```python
from build123d import *

# Parameters (mm, degrees)
SKETCH_1_R           = 1.7
EXTRUDE_1_DEPTH      = 4
EXTRUDE_2_DEPTH      = 4
EXTRUDE_2_DEPTH_BACK = 4


with BuildPart() as part:
    # Sketch 1 → Extrude 1 (new body)
    with BuildSketch(Plane(origin=(0, 0, 0), x_dir=(1, 0, 0), z_dir=(0, 1, 0))):
        with BuildLine():
            Line((0, -50), (0, -43))
            add(Edge.make_bspline(
                [(-10.000145873, 27.475174978), (-27.697978685, -43), (0, -43)],
                knots=[4.019246634, 4.019246634, 4.019246634, 6.283185307, 6.283185307, 6.283185307], degree=2, weights=[1, 0.42487789, 1]))
            ThreePointArc((-10.000145873, 27.475174978), (-18.360814479, 27.113576543), (-26.230013338, 24.266254592))
            add(Edge.make_bspline(
                [(-26.230013338, 24.266254592), (-50.964235719, -50), (0, -50)],
                knots=[4.205654034, 4.205654034, 4.205654034, 6.283185307, 6.283185307, 6.283185307], degree=2, weights=[1, 0.507284392, 1]))
        make_face()
        with Locations(Location((-3.997292475, -45.689262056, 0), (0, 0, 270))):
            Circle(SKETCH_1_R, mode=Mode.SUBTRACT)
        with Locations(Location((-21.5, 0, 0), (0, 0, 270))):
            Circle(SKETCH_1_R, mode=Mode.SUBTRACT)
    extrude(amount=EXTRUDE_1_DEPTH)

    # Sketch 2 → Extrude 2 (add, two sides: drawn at the far end of the back side and taken through both)
    with BuildSketch(Plane(origin=(0, 4, 0), x_dir=(1, 0, 0), z_dir=(0, 1, 0)).offset(-EXTRUDE_2_DEPTH_BACK)):
        with BuildLine():
            Line((0, -38), (0, -43))
            add(Edge.make_bspline(
                [(-10.438251501, 27.444344811), (-37.035399945, -43), (0, -43)],
                knots=[3.911241966, 3.911241966, 3.911241966, 6.283185307, 6.283185307, 6.283185307], degree=2, weights=[1, 0.375396623, 1]))
            ThreePointArc((-10.438251501, 27.444344811), (-8.2192487, 27.171324469), (-6.029573118, 26.71984426))
            add(Edge.make_bspline(
                [(-6.029573118, 26.71984426), (-29.815932514, -38), (0, -38)],
                knots=[3.788795549, 3.788795549, 3.788795549, 6.283185307, 6.283185307, 6.283185307], degree=2, weights=[1, 0.317983135, 1]))
        make_face()
    extrude(amount=EXTRUDE_2_DEPTH + EXTRUDE_2_DEPTH_BACK)


solid = part.part
```
Geometry: final body of the model. Coordinates: model frame, mm. Give positions to 0.01 mm unless a question says otherwise; leave off trailing zeros.
1. Section query A-A, the plane y = 2.75. Count the separate pieces of the cut face and the enclosed holes in it, then the cut area to 3 significant figures.
2. Draft query along Z for faces 1 (the flat face through (-20, 4, 8)), 2 (the cylindrical face through (-3.49, 1.97, 47.31)), 3 (the cylindrical face through (-18.245, 1.972, -27.136)). Return one class per face: released by +Z, released by -Z, zero draft, split by the parting line, or undercut.
3. Line query: probe 1 along Y at (x, z) = (-26, -18); probe 2 along X at (y, z) = (2, 0); probe 3 along X at (y, z) = (3, -0.5). Output: solid intervals per line, ascending.
4. Pin query (flat end, axial travel): P1, Ø2, axis at y = 2, z = 26, coming from the -X side; P2, Ø1.5, axis at y = 4, z = 29, coming from the -X side; P3, Ø4, axis at y = 4.5, z = 5, coming from the +X side. Return the tip coordinate at first contact, or that it passes through.
Computed:
1. separate pieces: 1
1. enclosed holes: 2
1. area: 1,390 mm2
2. face 1: zero draft
2. face 2: undercut
2. face 3: released by -Z
3. probe 1: y = 0 to 4
3. probe 2: x = -30 to -23.2, -19.8 to -9.98
3. probe 3: x = -30 to -23.12, -19.88 to -9.98
4. P1: stops at x = -25.98
4. P2: stops at x = -24.75
4. P3: stops at x = -9.9
